from build123d import *

# Parameters (mm, degrees)
F0_W     = 108
F0_H     = 65
F1_DEPTH = 25
F2_R     = 2.99999


# Not quite as in the source:
# - a fillet or chamfer is up to 0.001 mm smaller than in the source, because OpenCascade refuses the exact size


with BuildPart() as f1:
    # F0 (on Top) → F1 (new body)
    with BuildSketch(Plane.XY):
        Polygon((60.0555262864, 38.5), (-60.0555262864, 38.5), (-65, 33.5555262864), (-65, -33.5555262864), (-60.0555262864, -38.5), (60.0555262864, -38.5), (65, -33.5555262864), (65, 33.5555262864), align=None)
        Rectangle(F0_W, F0_H, mode=Mode.SUBTRACT)
    extrude(amount=F1_DEPTH)

    # F2 (radius 3 in the source; OpenCascade refuses exactly that, so slightly less here)
    f2_edges = [f1.edges().sort_by_distance(p)[0] for p in [
        (65, 0, 25),
        (62.527763, 36.027763, 25),
        (0, 38.5, 25),
        (-62.527763, 36.027763, 25),
        (-65, 0, 25),
        (-62.527763, -36.027763, 25),
        (0, -38.5, 25),
        (62.527763, -36.027763, 25),
        (-54, 0, 25),
        (0, 32.5, 25),
        (54, 0, 25),
        (0, -32.5, 25),
    ]]
    fillet(f2_edges, radius=F2_R)


solid = f1.part
Design review of the part built by this model. Coordinates are the model's own, in mm. A direction names the side the tool comes from. Coordinates: 2 decimals unless noted, no trailing zeros. Order: outer loops, then holes, each group sorted by start corner. A loop starts at its lowest first (then second) coordinate and runs counter-clockwise, first axis right, second up. Notation, with made-up numbers: (19, 23.5) - (40, 23.5) arc R23 cw to (40, 53.5) - close; hole circle Ø8 at (-31.75, 3). An arc over 180 degrees is marked (long way). Put each result on its own line as item: value.
1) Take a section at B-B, the plane z = 14.25. Give the boundary of the cut face in (x, y), and give its area (3 significant figures).
Response values:
outline: (-65, -33.56) - (-60.06, -38.5) - (60.06, -38.5) - (65, -33.56) - (65, 33.56) - (60.06, 38.5) - (-60.06, 38.5) - (-65, 33.56) - close; hole (-54, -32.5) - (54, -32.5) - (54, 32.5) - (-54, 32.5) - close
area: 2,940 mm²
2) The part is to be moulded in two halves that separate along Y. For faces 1 (the face through (-1, -38.5, 11)), 2 (the face through (62.562, 35.993, 10.846)), 3 (the face through (-1, -32.5, 11)), say which applies: released by +Y, released by -Y, zero draft, split by the parting line, or undercut.
Response values:
face 1: released by -Y
face 2: released by +Y
face 3: undercut
3) Tool access review of faces 4 (the face through (54, 0, 11)), 5 (the face through (0.8, -33.36, 24.1)), 6 (the face through (1, 38.5, 11)): name each direction out of +Z, -Z, +X, -X, +Y, -Y from which nothing blocks a thin tool from reaching the whole face with its end or side.
Response values:
face 4: +Z, -Z
face 5: +Z
face 6: +Z, -Z, +X, -X, +Y
4) Take a section at C-C, the plane y = -20. Give the boundary of the cut face in (x, z), and give its area (3 significant figures).
Response values:
outline: (-65, 0) - (-54, 0) - (-54, 22) arc R3 ccw to (-57, 25) - (-62, 25) arc R3 ccw to (-65, 22) - close; (54, 0) - (65, 0) - (65, 22) arc R3 ccw to (62, 25) - (57, 25) arc R3 ccw to (54, 22) - close
area: 542 mm²
5) Wall thickness on L1, parallel to X at y = -22.5, z = 21; L2, parallel to Y at x = -35, z = 17.25; L3, parallel to X at y = -35, z = 16.5: over which ranges is each line inside the solid? List them lowest first. Write a range as from..to.
Response values:
L1: x = -65..-54, 54..65
L2: y = -38.5..-32.5, 32.5..38.5
L3: x = -63.56..63.56
